CAD build for the part. Positions are in the model's coordinates, mm. Give positions to 0.01 mm unless a question says otherwise; leave off trailing zeros. Loops run counter-clockwise (first coordinate to the right, second up) from the corner with the lowest first, then second, coordinate; pieces in that order, holes last. Notation, with made-up numbers: (-28.75, 24.25) - (-6.75, 24.25) arc R26 cw to (-6.75, 38.25) - close; hole circle Ø8 at (53, 28). An arc over 180 degrees is marked (long way). Return JSON: item names as keys, results as strings.
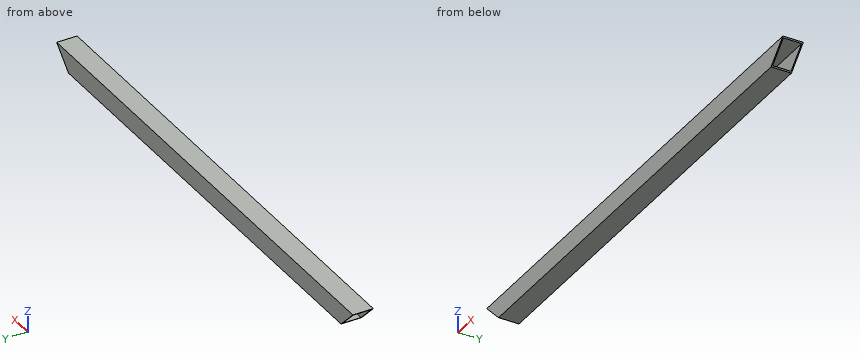
from build123d import *

# Parameters (mm, degrees)
CROQUIS1_W              = 40
CROQUIS1_H              = 40
CROQUIS1_W_2            = 36
CROQUIS1_H_2            = 36
SALIENTE_EXTRUIR1_DEPTH = 1000
CORTAR_EXTRUIR1_DEPTH   = 41


with BuildPart() as part:
    # Croquis1 → Saliente-Extruir1 (new body)
    with BuildSketch(Plane(origin=(0, 0, 0), x_dir=(0, 0, -1), z_dir=(1, 0, 0))):
        Rectangle(CROQUIS1_W, CROQUIS1_H)
        Rectangle(CROQUIS1_W_2, CROQUIS1_H_2, mode=Mode.SUBTRACT)
    extrude(amount=SALIENTE_EXTRUIR1_DEPTH)

    # Croquis2 → Cortar-Extruir1 (cut, through all)
    with BuildSketch(Plane(origin=(0, 20, 0), x_dir=(1, 0, 0), z_dir=(0, 1, 0))):
        Polygon((0, -20), (40, 20), (0, 20), align=None)
        Polygon((1000, 20), (1000, -20), (960, 20), align=None)
    extrude(amount=-CORTAR_EXTRUIR1_DEPTH, mode=Mode.SUBTRACT)


solid = part.part
1. Drop a flat-ended pin along its axis: P1, Ø10, axis at y = -13.5, z = -3.5, coming from the +X side. Give the stop position or say it passes through.
Values follow:
{"P1": "stops at x = 978.68"}
2. Cut at C-C, the plane x = 456. Write the cut outline in (y, z), plus the area to 3 significant figures.
Values follow:
{"outline": "(-20, -20) - (20, -20) - (20, 20) - (-20, 20) - close; hole (-18, -18) - (18, -18) - (18, 18) - (-18, 18) - close", "area": "304 mm²"}
3. Cut at B-B, the plane y = -1.5. Write the cut outline in (x, z).
Values follow:
{"outline": "(0, 20) - (2, 18) - (998, 18) - (1000, 20) - close; (38, -18) - (40, -20) - (960, -20) - (962, -18) - close"}
4. Cut at A-A, the plane z = 6.5. Write the cut outline in (x, y).
Values follow:
{"outline": "(13.5, -20) - (986.5, -20) - (986.5, -18) - (13.5, -18) - close; (13.5, 18) - (986.5, 18) - (986.5, 20) - (13.5, 20) - close"}
5. Drill centre line: probe 1 along Z at (x, y) = (636, -12.5). Where is it in solid material? Low to high.
Values follow:
{"probe 1": "z = -20 to -18, 18 to 20"}
